from build123d import *

# Parameters (mm, degrees)
CONG_1_R                                           = 2
CHANFREIN1_SIZE                                    = 0.5
ENL_V_MAT_EXTRU_1_DEPTH                            = 4
TROU_TARAUD_M41_D                                  = 3.3
CHAMBRAGE_POUR_VIS_T_TE_HEXAGONALE_M41_D           = 4.3
CHAMBRAGE_POUR_VIS_T_TE_HEXAGONALE_M41_CBORE_D     = 8
CHAMBRAGE_POUR_VIS_T_TE_HEXAGONALE_M41_CBORE_DEPTH = 5
CHANFREIN2_SIZE                                    = 0.2
TROU_TARAUD_M31_D                                  = 2.5
TROU_TARAUD_M31_CSINK_D                            = 4.5
TROU_TARAUD_M31_CSINK_ANGLE                        = 90


with BuildPart() as part:
    # Esquisse1 → Révolution1 (revolve)
    with BuildSketch(Plane.XY, mode=Mode.PRIVATE) as r_volution1_sk:
        Polygon((0, 55), (0, 65), (13, 65), (13, 55), (14, 55), (14, 43), (4, 43), (4, 55), align=None)
    revolve(r_volution1_sk.sketch.rotate(Axis((0, 0, 0), (1, 0, 0)), 90), axis=Axis((0, 0, 0), (1, 0, 0)))

    # Congé1
    cong_1_edges = [part.edges().sort_by_distance(p)[0] for p in [
        (0, 0, -65),
    ]]
    fillet(cong_1_edges, radius=CONG_1_R)

    # Chanfrein1
    chanfrein1_edges = [part.edges().sort_by_distance(p)[0] for p in [
        (0, 0, -55),
    ]]
    chamfer(chanfrein1_edges, length=CHANFREIN1_SIZE)

    # Esquisse5 → Enlèv. mat.-Extru.1 (cut)
    with BuildSketch(Plane.ZY):
        Polygon((-5, 80), (-5, 5), (-80, 5), (-80, -5), (-5, -5), (-5, -80), (5, -80), (5, -5), (5, 5), (5, 80), align=None)
    extrude(amount=-ENL_V_MAT_EXTRU_1_DEPTH, mode=Mode.SUBTRACT)

    # Trou taraudé M41 (through all)
    with Locations(Plane(origin=(14, 0, 0), x_dir=(0, 0, -1), z_dir=(1, 0, 0))):
        with Locations((0, 47.5), (47.5, 0), (0, -47.5), (-47.5, 0)):
            Hole(TROU_TARAUD_M41_D / 2)

    # Chambrage pour vis à tête hexagonale M41 (through all)
    with Locations(Plane(origin=(14, 0, 0), x_dir=(0, 0, -1), z_dir=(1, 0, 0))):
        with Locations((0, 60), (60, 0), (0, -60)):
            CounterBoreHole(CHAMBRAGE_POUR_VIS_T_TE_HEXAGONALE_M41_D / 2, CHAMBRAGE_POUR_VIS_T_TE_HEXAGONALE_M41_CBORE_D / 2, CHAMBRAGE_POUR_VIS_T_TE_HEXAGONALE_M41_CBORE_DEPTH)

    # Chanfrein2
    chanfrein2_edges = [part.edges().sort_by_distance(p)[0] for p in [
        (14, 0, -55),
    ]]
    chamfer(chanfrein2_edges, length=CHANFREIN2_SIZE)

    # Trou taraudé M31 (through all)
    with Locations(Plane(origin=(13, 0, 0), x_dir=(0, 0, -1), z_dir=(1, 0, 0))):
        with Locations((42.426406871, 42.426406871), (42.426406871, -42.426406871), (-42.426406871, -42.426406871), (-42.426406871, 42.426406871)):
            CounterSinkHole(TROU_TARAUD_M31_D / 2, TROU_TARAUD_M31_CSINK_D / 2, counter_sink_angle=TROU_TARAUD_M31_CSINK_ANGLE)


solid = part.part
Source: CAD feature listing. Evaluate the final solid. Frame: model axes, mm. A direction names the side the tool comes from. Give positions to 0.01 mm unless a question says otherwise; leave off trailing zeros. Return JSON: item names as keys, results as strings. Group by question number.
1. Access query for faces 4 (the face through (2, -5, -60)), 5 (the face through (8.93, 0.07, -49.15)), 6 (the face through (0, -38, -42)), 7 (the face through (4, -14, -41)), 8 (the face through (11.028, -63.905, 0.867)). Directions: +Z, -Z, +X, -X, +Y, -Y. A direction counts if a zero-diameter tool reaches every point of the face in a straight line with its end or side. Return the directions, or none.
2. Pin query (flat end, axial travel): pin 1 Ø5.5 at (y, z) = (-47.5, 0) entering from +X; pin 2 Ø6.5 at (y, z) = (-0.5, -60) entering from +X; pin 3 Ø2 at (x, y) = (11.5, 10) entering from +Z; pin 4 Ø4.5 at (x, z) = (1, -61) entering from +Y. Return the tip coordinate at first contact, or that it passes through.
3. Section A-A, the plane y = 0. Count the separate pieces of the cut face and the enclosed holes in it, then the cut area to 3 significant figures.
4. Material intervals for line 1 (Y direction, x = 9.75, z = 0); line 2 (Y direction, x = 6.75, z = 0); line 3 (X direction, y = -17.5, z = 39.5), sorted ascending. Write a range as from..to.
5. Mould query, pull axis Y, two halves, no side actions, for faces 1 (the face through (11.028, 56.095, 0.867)), 2 (the face through (13.406, 48.794, 25.379)), 3 (the face through (0, 40, -40)). Classes: +Y half, -Y half, draft (parallel to the pull), parting line (faces both ways), or undercut.
Determined:
{
 "1": {"face 4": "-Z, -X", "face 5": "+X, -X", "face 6": "+Z, -Z, -X, +Y, -Y", "face 7": "-X", "face 8": "+X"},
 "2": {"pin 1": "stops at x = 14", "pin 2": "stops at x = 9", "pin 3": "stops at z = 64.37", "pin 4": "stops at y = 27.55"},
 "3": {"separate pieces": "5", "enclosed holes": "0", "area": "339 mm2"},
 "4": {"line 1": "y = -65..-64, -56..-49.15, -45.85..-43, 43..45.85, 49.15..56, 64..65", "line 2": "y = -65..-62.15, -57.85..-49.15, -45.85..-43, 43..45.85, 49.15..57.85, 62.15..65", "line 3": "x = 4..14"},
 "5": {"face 1": "undercut", "face 2": "parting line", "face 3": "draft"}
}
